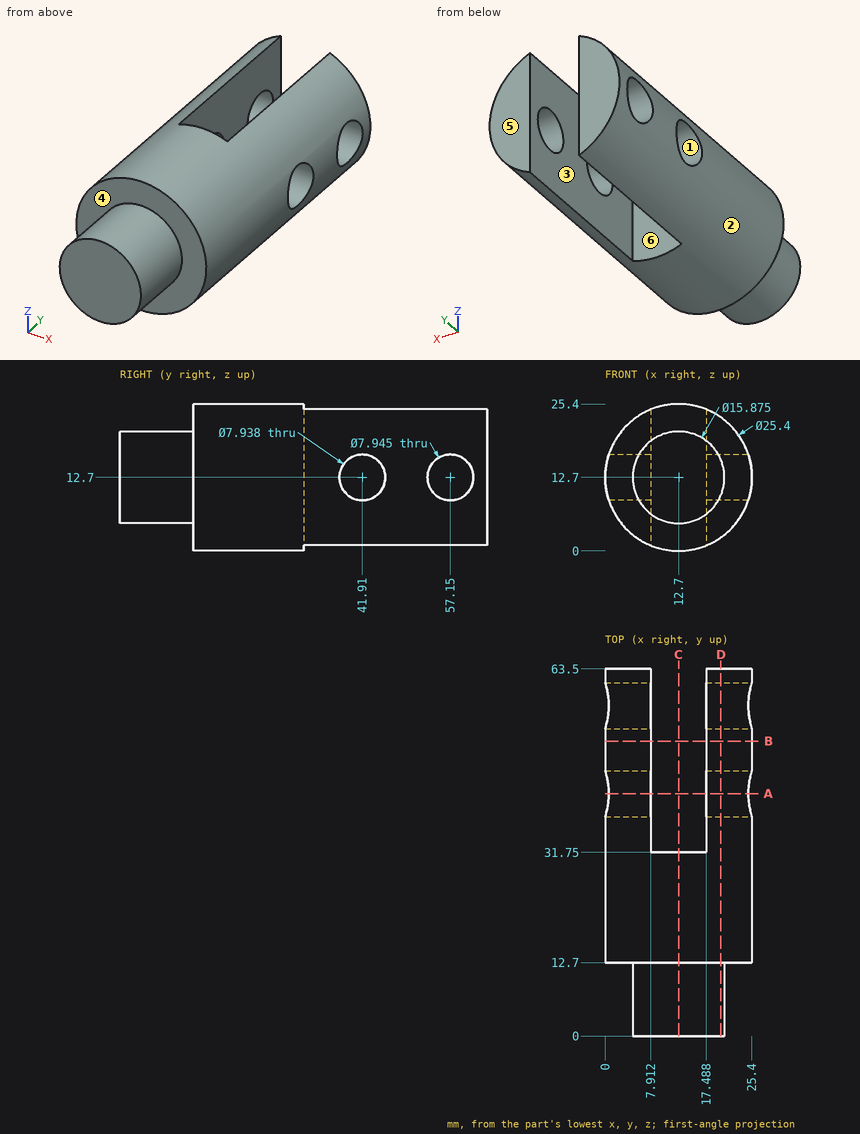
Here's the drawing with two shaded views (mm, measured from the low corner). I have some questions. A direction names the side the tool comes from. Coordinates: 2 decimals unless noted, no trailing zeros. Order: outer loops, then holes, each group sorted by start corner. A loop starts at its lowest first (then second) coordinate and runs counter-clockwise, first axis right, second up.
Q1. Suppose I cut it at B-B on y = 51. Please give me the cut outline in (x, z), and give its area (3 significant figures).
Q2. Which directions (+Z, -Z, +X, -X, +Y, -Y) give clear straight access to the entire face, cutting with the end or side of a thin tool? Please do the marked faces 4, 5 and 6.
Q3. Will these pins go through, and if not, where does the flat tip stop? pin 1 (4 mm diameter, centred on y = 54.5, z = 10.5, fed in from -X); pin 2 (6 mm diameter, centred on y = 38.5, z = 21, fed in from -X); pin 3 (6.5 mm diameter, centred on y = 41.91, z = 12.7, fed in from -X); pin 4 (2 mm diameter, centred on x = 5.5, y = 50, fed in from -Z) (1 decimal).
Q4. Suppose I cut it at A-A on y = 41.91. Please give me the cut outline in (x, z), and give its area (3 significant figures).
Q5. Suppose I cut it at D-D on x = 20. Give the number of separate pieces and of enclosed holes in the cut face, and give its area (3 significant figures).
Q6. Suppose I cut it at C-C on x = 12.7. Please give me the cut outline in (y, z).
Q7. Please list where these lines run through material, in increasing order: L1, parallel to Y at x = 20.5, z = 12.7; L2, parallel to Y at x = 2.5, z = 12.7; L3, parallel to X at y = 33.5, z = 12.25.
Q8. Thinking about a two-plate mould opening in Z: for the marked faces 1, 2 and 3, which applies, released by +Z, released by -Z, zero draft, split by the parting line, or undercut?
Answer:
1. outline: (7.91, 0.94) - (7.91, 24.46) arc R12.7 ccw to start; (17.49, 0.94) arc R12.7 ccw to (17.49, 24.46) - close
1. area: 269 mm2
2. face 4: -Y
2. face 5: +Z, -Z, +X, -X, +Y
2. face 6: +Z, -Z, +Y
3. pin 1: stops at x = 0.02
3. pin 2: stops at x = 1.16
3. pin 3: passes through
3. pin 4: stops at z = 1.6
4. outline: (0.64, 8.73) arc R12.7 ccw to (7.91, 0.94) - (7.91, 8.73) - close; (0.64, 16.67) - (7.91, 16.67) - (7.91, 24.46) arc R12.7 ccw to start; (17.49, 0.94) arc R12.7 ccw to (24.76, 8.73) - (17.49, 8.73) - close; (17.49, 16.67) - (24.76, 16.67) arc R12.7 ccw to (17.49, 24.46) - close
4. area: 147 mm2
5. separate pieces: 1
5. enclosed holes: 2
5. area: 1,040 mm2
6. outline: (0, 4.76) - (12.7, 4.76) - (12.7, 0) - (31.75, 0) - (31.75, 25.4) - (12.7, 25.4) - (12.7, 20.64) - (0, 20.64) - close
7. L1: y = 0 to 37.94, 45.88 to 53.18, 61.12 to 63.5
7. L2: y = 12.7 to 37.94, 45.88 to 53.18, 61.12 to 63.5
7. L3: x = 0.01 to 7.91, 17.49 to 25.39
8. face 1: undercut
8. face 2: split by the parting line
8. face 3: zero draft
